Work out the finished part from the listing and answer in its coordinate system (mm). Face numbers are marked on the shaded views. A direction names the side the tool comes from. Give positions to 0.01 mm unless a question says otherwise; leave off trailing zeros. Order: outer loops, then holes, each group sorted by start corner. A loop starts at its lowest first (then second) coordinate and runs counter-clockwise, first axis right, second up. Notation, with made-up numbers: (85, -16.75) -> (110, -16.75) arc R24 ccw to (110, 10.25) -> close; hole circle Ø3 at (20.5, 26.25). An arc over 180 degrees is marked (long way). Use a Markdown table: item, result. Add a question column.
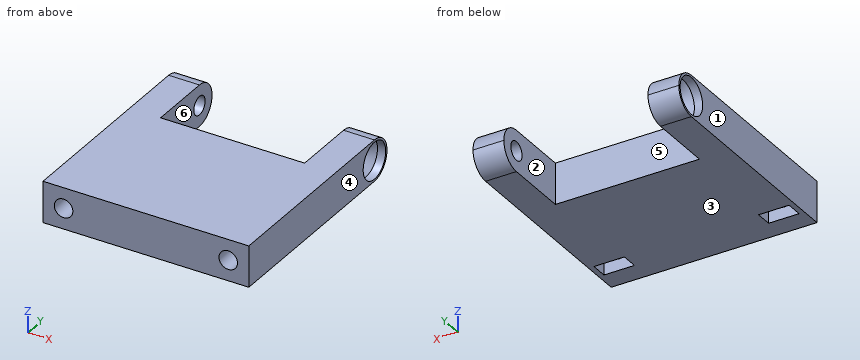
```python
from build123d import *

# Parameters (mm, degrees)
SKETCH1_W                = 50
SKETCH1_H                = 10
BOSS_EXTRUDE1_DEPTH      = 55
FILLET1_R                = 5
SKETCH2_W                = 35
SKETCH2_H                = 20.5
CUT_EXTRUDE1_DEPTH       = 62.23724357
M4_CLEARANCE_HOLE1_D     = 4.5
M4_CLEARANCE_HOLE1_DEPTH = 9
M4_CLEARANCE_HOLE1_TIP   = 1.351936393
SKETCH9_W                = 7.4
SKETCH9_H                = 4
CUT_EXTRUDE2_DEPTH       = 9


with BuildPart() as part:
    # Sketch1 → Boss-Extrude1 (new body)
    with BuildSketch(Plane(origin=(0, 0, 0), x_dir=(1, 0, 0), z_dir=(0, 1, 0))):
        Rectangle(SKETCH1_W, SKETCH1_H)
    extrude(amount=BOSS_EXTRUDE1_DEPTH)

    # Fillet1
    fillet1_edges = [part.edges().sort_by_distance(p)[0] for p in [
        (0, 55, -5),
        (0, 55, 5),
    ]]
    fillet(fillet1_edges, radius=FILLET1_R - 0.0001)  # a hair under: the kernel refuses the full size

    # Sketch2 → Cut-Extrude1 (cut, through all)
    with BuildSketch(Plane.XY.offset(5)):
        with Locations((0, 44.75)):
            Rectangle(SKETCH2_W, SKETCH2_H)
    extrude(amount=-CUT_EXTRUDE1_DEPTH, mode=Mode.SUBTRACT)

    # Sketch5 → CSK for M4 SFHCS1 (revolve, cut)
    with BuildSketch(Plane(origin=(-25, 50, 0), x_dir=(0, 0, 1), z_dir=(0, 1, 0))):
        Polygon((0, 0), (0, 50), (2.25, 50), (2.25, 4.23), (4.48, 2), (4.48, 0), align=None)
    csk_for_m4_sfhcs1 = revolve(axis=Axis((-31.35, 50, 0), (1, 0, 0)), mode=Mode.SUBTRACT)

    # Mirror1: CSK for M4 SFHCS1 across plane
    add(csk_for_m4_sfhcs1.mirror(Plane(origin=(0, 0, 0), x_dir=(0, 0, 1), z_dir=(1, 0, 0))), mode=Mode.SUBTRACT)

    # M4 Clearance Hole1
    with Locations(Plane(origin=(0, 0, 0), x_dir=(-1, 0, 0), z_dir=(0, -1, 0))):
        with Locations((-20, 0), (20, 0)):
            Hole(M4_CLEARANCE_HOLE1_D / 2, depth=M4_CLEARANCE_HOLE1_DEPTH)
            with Locations((0, 0, -(M4_CLEARANCE_HOLE1_DEPTH + M4_CLEARANCE_HOLE1_TIP / 2))):  # 118° drill point
                Cone(0, M4_CLEARANCE_HOLE1_D / 2, M4_CLEARANCE_HOLE1_TIP, mode=Mode.SUBTRACT)

    # Sketch9 → Cut-Extrude2 (cut)
    with BuildSketch(Plane(origin=(0, 0, -5), x_dir=(-1, 0, 0), z_dir=(0, 0, -1))):
        with Locations((20, 7)):
            Rectangle(SKETCH9_W, SKETCH9_H)
    cut_extrude2 = extrude(amount=-CUT_EXTRUDE2_DEPTH, mode=Mode.SUBTRACT)

    # Mirror2: Cut-Extrude2 across plane
    add(cut_extrude2.mirror(Plane(origin=(0, 0, 0), x_dir=(0, 0, 1), z_dir=(1, 0, 0))), mode=Mode.SUBTRACT)


solid = part.part
```
1) Which of the six approach directions +Z, -Z, +X, -X, +Y, -Y give full straight-line access (tool end or side, diameter ignored) to the marked faces 1 and 2?
2) The part is cut by section B-B, the plane x = 15. Determine the outline of the cut face in (y, z), then the cut area to 3 significant figures.
3) Determine the mould class of the marked faces 3, 4, 5 and 6 for opening direction X: released by +X, released by -X, zero draft, split by the parting line, or undercut.
4) The part is cut by section A-A, the plane y = 38.5. Determine the outline of the cut face in (x, z).
5) Flat-ended cylindrical pins translate along their axes: pin 1 (2 mm diameter, centred on x = 20.5, z = -0.5, fed in from +Y); pin 2 (2 mm diameter, centred on x = -20, y = 7.5, fed in from -Z); pin 3 (1.5 mm diameter, centred on x = -15.5, z = 2, fed in from +Y); pin 4 (5 mm diameter, centred on y = 50, z = 0, fed in from +X). Find the tip coordinate at first contact, or state that the pin passes through.
6) The part is cut by section C-C, the plane z = -1.25. State how many separate pieces and enclosed holes the cut face has, then the cut area to 3 significant figures.
7) Straight lines are drawn through the part: line 1 (Z direction, x = -19.8, y = 50); line 2 (X direction, y = 36, z = 3); line 3 (Z direction, x = 23, y = 50). For each, find the intervals that lie inside material, in ascending order.
A:
| question | item | result |
|---|---|---|
| 1 | face 1 | +Z, -Z, -X, +Y, -Y |
| 1 | face 2 | +Z, -Z, +Y |
| 2 | outline | (0, -5) -> (34.5, -5) -> (34.5, 5) -> (0, 5) -> close |
| 2 | area | 345 mm^2 |
| 3 | face 3 | zero draft |
| 3 | face 4 | released by +X |
| 3 | face 5 | undercut |
| 3 | face 6 | undercut |
| 4 | outline | (-25, -5) -> (-17.5, -5) -> (-17.5, 5) -> (-25, 5) -> close; (17.5, -5) -> (25, -5) -> (25, 5) -> (17.5, 5) -> close |
| 5 | pin 1 | y = 55 |
| 5 | pin 2 | z = 4 |
| 5 | pin 3 | y = 34.5 |
| 5 | pin 4 | x = 21.02 |
| 6 | separate pieces | 3 |
| 6 | enclosed holes | 0 |
| 6 | area | 1,840 mm^2 |
| 7 | line 1 | -5 to -2.25, 2.25 to 5 |
| 7 | line 2 | -25 to -17.5, 17.5 to 25 |
| 7 | line 3 | -5 to -4.48, 4.48 to 5 |
